Source: CAD feature listing. Evaluate the final solid. Frame: model axes, mm. Face numbers are marked on the shaded views. A direction names the side the tool comes from. Coordinates: 2 decimals unless noted, no trailing zeros. Write each loop counter-clockwise with the first axis right and the second up, starting at its lowest first coordinate (ties: lowest second). Pieces come first, ordered by that corner, then holes. Notation, with made-up numbers: M 28.5,50 L 83.5,50 A15 cw 83.5,79 Z; hole C 75.25,71 d9. An arc over 180 degrees is marked long. Write item = value, one per line. Start each with the question number.
1. Section query C-C (z = 9.75). Output: boundary loops of the cut face in (x, y).
2. Section query B-B (x = -0.2). Output: boundary loops of the cut face in (y, z), then the cut area to 3 significant figures.
3. Pull-direction query (Z, two-part tool) for the marked faces 1, 2 and 3; classes: pulls with the +Z half, pulls with the -Z half, needs draft (parallel to the pull), parting line crosses it, or undercut.
4. Section query D-D (y = -20.25). Output: boundary loops of the cut face in (x, z), then the cut area to 3 significant figures.
5. Section query A-A (y = -13). Output: boundary loops of the cut face in (x, z).
6. Pin query (flat end, axial travel): pin 1 Ø3 at (x, z) = (-8, 22.5) entering from -Y; pin 2 Ø1.5 at (x, y) = (5.5, -21) entering from +Z. Return the tip coordinate at first contact, or that it passes through.
7. Access query for the marked faces 4, 5 and 6. Directions: +Z, -Z, +X, -X, +Y, -Y. A direction counts if a zero-diameter tool reaches every point of the face in a straight line with its end or side. Return the directions, or none.
8. Line query: line 1 along X through (y, z) = (-5, 6.25); line 2 along Y through (x, z) = (0, 3); line 3 along Z through (x, y) = (-4, -7.5). Output: solid intervals per line, ascending.
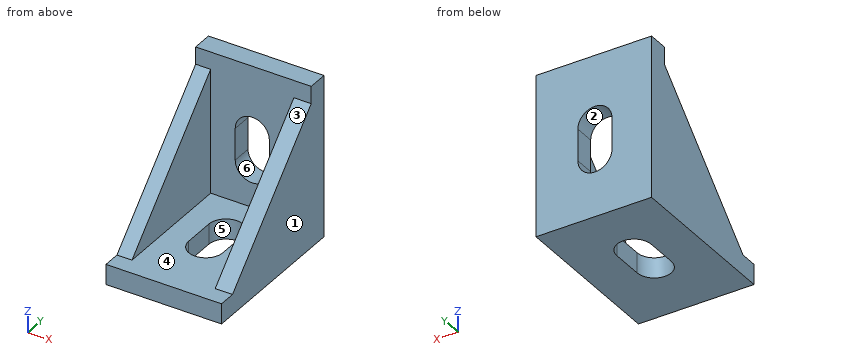
```python
from build123d import *

# Parameters (mm, degrees)
PAD_DEPTH            = 10
BOX_W                = 27
BOX_H                = 24.4
BOX_DEPTH            = 14.4
POCKET_DEPTH         = 3.5
POCKET001_DEPTH      = 4
BODY_ROLL_ANGLE      = 90
BODY_PLACEMENT_ANGLE = -90


with BuildPart() as part:
    # Sketch → Pad (new body, symmetric)
    with BuildSketch(Plane.XY):
        Polygon((0, 0), (0, 28), (3.5, 28), (3.5, 25), (25, 3.5), (28, 3.5), (28, 0), align=None)
    extrude(amount=PAD_DEPTH, both=True)

    # Box → Box (cut)
    with BuildSketch(Plane(origin=(3.5, 3.5, -7), x_dir=(1, 0, 0), z_dir=(0, 0, 1))):
        with Locations((13.5, 12.2)):
            Rectangle(BOX_W, BOX_H)
    extrude(amount=BOX_DEPTH, mode=Mode.SUBTRACT)

    # Sketch001 (on Face17 of Box) → Pocket (cut)
    with BuildSketch(Plane(origin=(3.5, 3.5, -7), x_dir=(0, 1, 0), z_dir=(1, 0, 0))):
        with BuildLine():
            ThreePointArc((7.2, 10.15), (4.25, 7.2), (7.2, 4.25))
            Line((7.2, 4.25), (12.7, 4.25))
            ThreePointArc((12.7, 4.25), (15.65, 7.2), (12.7, 10.15))
            Line((7.2, 10.15), (12.7, 10.15))
        make_face()
    extrude(amount=-POCKET_DEPTH, mode=Mode.SUBTRACT)

    # Sketch002 (on Face21 of Pocket) → Pocket001 (cut)
    with BuildSketch(Plane(origin=(3.5, 3.5, -7), x_dir=(-1, 0, 0), z_dir=(0, 1, 0))):
        with BuildLine():
            ThreePointArc((-12.7, 10.15), (-15.65, 7.2), (-12.7, 4.25))
            Line((-12.7, 4.25), (-7.2, 4.25))
            ThreePointArc((-7.2, 4.25), (-4.25, 7.2), (-7.2, 10.15))
            Line((-12.7, 10.15), (-7.2, 10.15))
        make_face()
    extrude(amount=-POCKET001_DEPTH, mode=Mode.SUBTRACT)


with BuildPart() as part_1:
    # Body roll: moved
    add(part.part.rotate(Axis((0, 0, 0), (1, 0, 0)), BODY_ROLL_ANGLE))


with BuildPart() as part_2:
    # Body placement: moved
    add(part_1.part.rotate(Axis((0, 0, 0), (0, 0, 1)), BODY_PLACEMENT_ANGLE))


solid = part_2.part
```
Results are:
q1.outline = M -10,-18.75 L -7.4,-18.75 L -7.4,-3.5 L -2.99,-3.5 L -2.99,0 L -10,0 Z; M 2.59,-3.5 L 7,-3.5 L 7,-18.75 L 10,-18.75 L 10,0 L 2.59,0 Z
q2.outline = M -28,0 L -19.15,0 L -19.15,3.5 L -28,3.5 Z; M -7.75,0 L 0,0 L 0,7.75 L -3.5,7.75 L -3.5,3.5 L -7.75,3.5 Z; M -3.5,19.15 L 0,19.15 L 0,28 L -3.5,28 Z
q2.area = 104 mm^2
q3.face_1 = needs draft
q3.face_2 = undercut
q3.face_3 = pulls with the +Z half
q4.outline = M -10,0 L 10,0 L 10,8.25 L 7,8.25 L 7,3.5 L -7.4,3.5 L -7.4,8.25 L -10,8.25 Z
q4.area = 96.6 mm^2
q5.outline = M -10,0 L -3.15,0 L -3.15,3.5 L -7.4,3.5 L -7.4,15.5 L -10,15.5 Z; M 2.75,0 L 10,0 L 10,15.5 L 7,15.5 L 7,3.5 L 2.75,3.5 Z
q6.pin_1 = -7.5
q6.pin_2 = 3.5
q7.face_4 = +Z, -Y
q7.face_5 = +Z, -Z
q7.face_6 = +Y, -Y
q8.line_1 = -10 to -7.4, 7 to 10
q8.line_2 = -28 to -19.14, -7.76 to 0
q8.line_3 = 0 to 3.5
